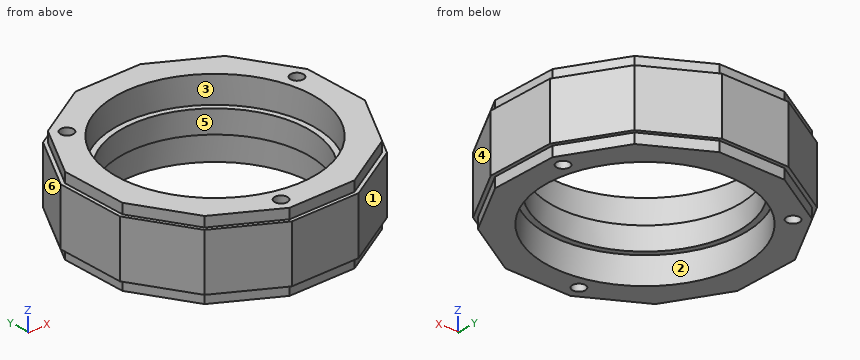
```python
from build123d import *

# Parameters (mm, degrees)
S01_SMALLER_TWELVE_FLAT_END_BEAD_SEATS_R      = 24.6
F_01_SMALLER_TWELVE_FLAT_END_BEAD_SEATS_DEPTH = 20.2
F_02_START                                    = 2.65
S02_RAISED_CENTRAL_TYRE_DRIVE_KEY_R           = 24.6
F_02_RAISED_CENTRAL_TYRE_DRIVE_KEY_DEPTH      = 14.9
F_03_START                                    = -0.1
S03_INBOARD_6808_OUTER_RACE_SEAT_R            = 26.1
F_03_INBOARD_6808_OUTER_RACE_SEAT_DEPTH       = 7.2
F_04_START                                    = 13.1
S04_OUTBOARD_6808_OUTER_RACE_SEAT_R           = 26.1
F_04_OUTBOARD_6808_OUTER_RACE_SEAT_DEPTH      = 7.2
F_05_START                                    = -0.1
S05_THREE_TYRE_FLANGE_THROUGH_HOLES_R         = 1.7
F_05_THREE_TYRE_FLANGE_THROUGH_HOLES_DEPTH    = 20.4


with BuildPart() as part:
    # S01 - Smaller twelve-flat end bead seats → 01 - Smaller twelve-flat end bead seats (new body)
    with BuildSketch(Plane.XY):
        Polygon((32.551700346, 8.72220182), (23.829498526, 23.829498526), (8.72220182, 32.551700346), (-8.72220182, 32.551700346), (-23.829498526, 23.829498526), (-32.551700346, 8.72220182), (-32.551700346, -8.72220182), (-23.829498526, -23.829498526), (-8.72220182, -32.551700346), (8.72220182, -32.551700346), (23.829498526, -23.829498526), (32.551700346, -8.72220182), align=None)
        Circle(S01_SMALLER_TWELVE_FLAT_END_BEAD_SEATS_R, mode=Mode.SUBTRACT)
    extrude(amount=F_01_SMALLER_TWELVE_FLAT_END_BEAD_SEATS_DEPTH)

    # S02 - Raised central tyre drive key → 02 - Raised central tyre drive key (add)
    with BuildSketch(Plane.XY.offset(F_02_START)):
        Polygon((33.498307656, 8.975844484), (24.522463172, 24.522463172), (8.975844484, 33.498307656), (-8.975844484, 33.498307656), (-24.522463172, 24.522463172), (-33.498307656, 8.975844484), (-33.498307656, -8.975844484), (-24.522463172, -24.522463172), (-8.975844484, -33.498307656), (8.975844484, -33.498307656), (24.522463172, -24.522463172), (33.498307656, -8.975844484), align=None)
        Circle(S02_RAISED_CENTRAL_TYRE_DRIVE_KEY_R, mode=Mode.SUBTRACT)
    extrude(amount=F_02_RAISED_CENTRAL_TYRE_DRIVE_KEY_DEPTH)

    # S03 - Inboard 6808 outer race seat → 03 - Inboard 6808 outer race seat (cut)
    with BuildSketch(Plane.XY.offset(F_03_START)):
        Circle(S03_INBOARD_6808_OUTER_RACE_SEAT_R)
    extrude(amount=F_03_INBOARD_6808_OUTER_RACE_SEAT_DEPTH, mode=Mode.SUBTRACT)

    # S04 - Outboard 6808 outer race seat → 04 - Outboard 6808 outer race seat (cut)
    with BuildSketch(Plane.XY.offset(F_04_START)):
        Circle(S04_OUTBOARD_6808_OUTER_RACE_SEAT_R)
    extrude(amount=F_04_OUTBOARD_6808_OUTER_RACE_SEAT_DEPTH, mode=Mode.SUBTRACT)

    # S05 - Three tyre-flange through holes → 05 - Three tyre-flange through holes (cut)
    with BuildSketch(Plane.XY.offset(F_05_START)):
        with Locations((28.832885915, 7.725748496)):
            Circle(S05_THREE_TYRE_FLANGE_THROUGH_HOLES_R)
        with Locations((-21.107137418, 21.107137418)):
            Circle(S05_THREE_TYRE_FLANGE_THROUGH_HOLES_R)
        with Locations((-7.725748496, -28.832885915)):
            Circle(S05_THREE_TYRE_FLANGE_THROUGH_HOLES_R)
    extrude(amount=F_05_THREE_TYRE_FLANGE_THROUGH_HOLES_DEPTH, mode=Mode.SUBTRACT)


solid = part.part
```
Geometry check sheet. Reference: the model listing, model coordinates, mm. Face numbers are marked on the shaded views. A direction names the side the tool comes from. Give positions to 0.01 mm unless a question says otherwise; leave off trailing zeros. Order: outer loops, then holes, each group sorted by start corner. A loop starts at its lowest first (then second) coordinate and runs counter-clockwise, first axis right, second up. Notation, with made-up numbers: (-20, 38.5) - (10, 38.5) arc R30 ccw to (10, 60.5) - close; hole circle Ø10 at (76.5, -30.5). An arc over 180 degrees is marked (long way). Answer in a Markdown table with one row per item. Add a question column.
Q1. Cross-section at C-C, the plane z = 12.25. Enter the section's corners in (x, y).
Q2. Tool access check on the marked faces 1, 2 and 3. Record the directions out of +Z, -Z, +X, -X, +Y, -Y that give a thin tool (end or side, any length) a straight path to the whole face; none if there is none.
Q3. Material ranges on probe 1 along Y at (x, z) = (0, 9.55); probe 2 along X at (y, z) = (7, 10.25); probe 3 along Z at (x, y) = (-25.5, -22), recorded low to high. Write a range as from..to.
Q4. Cross-section at A-A, the plane y = 0. Enter the section's corners in (x, z), then the cut area to 3 significant figures.
Q5. Cross-section at D-D, the plane y = 29. Enter the section's corners in (x, z).
Q6. Mould release check, pull along X, two halves, no side actions. Record for the marked faces 4, 5 and 6: pulls with the +X half, pulls with the -X half, needs draft (parallel to the pull), parting line crosses it, or undercut.
Q7. Gauge pin test, flat ends, axial feed: pin 1 (0.8 mm diameter, centred on y = -4, z = 18.5, fed in from -X); pin 2 (2 mm diameter, centred on x = -3, z = 1.5, fed in from -Y); pin 3 (3 mm diameter, centred on x = 28.83, y = 7.73, fed in from -Z); pin 4 (3 mm diameter, centred on y = -23.5, z = 2, fed in from -X). Record the tip position at first contact, or that the pin passes through.
Check values:
| question | item | result |
|---|---|---|
| 1 | outline | (-33.5, -8.98) - (-24.52, -24.52) - (-8.98, -33.5) - (8.98, -33.5) - (24.52, -24.52) - (33.5, -8.98) - (33.5, 8.98) - (24.52, 24.52) - (8.98, 33.5) - (-8.98, 33.5) - (-24.52, 24.52) - (-33.5, 8.98) - close; hole circle Ø49.2 at (0, 0); hole circle Ø3.4 at (-21.11, 21.11); hole circle Ø3.4 at (-7.73, -28.83); hole circle Ø3.4 at (28.83, 7.73) |
| 2 | face 1 | +Z, -Z, +X, -Y |
| 2 | face 2 | -Z |
| 2 | face 3 | +Z |
| 3 | probe 1 | y = -33.5..-24.6, 24.6..33.5 |
| 3 | probe 2 | x = -33.5..-23.58, 23.58..27.3, 30.37..33.5 |
| 3 | probe 3 | z = 2.65..17.55 |
| 4 | outline | (-33.5, 2.65) - (-32.55, 2.65) - (-32.55, 0) - (-26.1, 0) - (-26.1, 7.1) - (-24.6, 7.1) - (-24.6, 13.1) - (-26.1, 13.1) - (-26.1, 20.2) - (-32.55, 20.2) - (-32.55, 17.55) - (-33.5, 17.55) - close; (24.6, 7.1) - (26.1, 7.1) - (26.1, 0) - (32.55, 0) - (32.55, 2.65) - (33.5, 2.65) - (33.5, 17.55) - (32.55, 17.55) - (32.55, 20.2) - (26.1, 20.2) - (26.1, 13.1) - (24.6, 13.1) - close |
| 4 | area | 307 mm^2 |
| 5 | outline | (-16.77, 2.65) - (-14.87, 2.65) - (-14.87, 0) - (14.87, 0) - (14.87, 2.65) - (16.77, 2.65) - (16.77, 17.55) - (14.87, 17.55) - (14.87, 20.2) - (-14.87, 20.2) - (-14.87, 17.55) - (-16.77, 17.55) - close |
| 6 | face 4 | pulls with the +X half |
| 6 | face 5 | undercut |
| 6 | face 6 | pulls with the -X half |
| 7 | pin 1 | stops at x = -32.55 |
| 7 | pin 2 | stops at y = -32.55 |
| 7 | pin 3 | passes through |
| 7 | pin 4 | stops at x = -25.89 |
